Source: CAD feature listing. Evaluate the final solid. Frame: model axes, mm. A direction names the side the tool comes from. Coordinates: 2 decimals unless noted, no trailing zeros. Loops run counter-clockwise (first coordinate to the right, second up) from the corner with the lowest first, then second, coordinate; pieces in that order, holes last. Notation, with made-up numbers: (21.5, 6) -> (48.5, 6) arc R18 cw to (48.5, 14) -> close; hole circle Ø10 at (-34.75, -34.75). An arc over 180 degrees is marked (long way). Answer as a JSON object with one key per item and string values. Group by question number.
from build123d import *

# Parameters (mm, degrees)
F1_DEPTH = 20
F2_T     = -3
F4_DEPTH = 20
F6_D     = 4.3
F6_DEPTH = 5
F6_TIP   = 1.2918503309


with BuildPart() as f1:
    # F0 (on Top) → F1 (new body)
    with BuildSketch(Plane.XY):
        Polygon((0, 100), (0, 0), (173.2050807569, 0), align=None)
    extrude(amount=F1_DEPTH)

    # F2
    f2_openings = [f1.faces().sort_by_distance(p)[0] for p in [
        (57.735027, 33.333333, 20),
        (57.735027, 33.333333, 0),
    ]]
    offset(amount=F2_T, openings=f2_openings)

    # F3 (on face) → F4 (join)
    with BuildSketch(Plane.XY.offset(20)):
        Polygon((86.6025403784, 3), (86.6025403784, 46.5358983849), (83.6025403784, 48.2679491924), (83.6025403784, 3), align=None)
    extrude(amount=-F4_DEPTH)

    # F6
    with Locations(Plane.XZ):
        with Locations((30, 10), (123.2050807569, 10)):
            Hole(F6_D / 2, depth=F6_DEPTH)
            with Locations((0, 0, -(F6_DEPTH + F6_TIP / 2))):  # 118° drill point
                Cone(0, F6_D / 2, F6_TIP, mode=Mode.SUBTRACT)


solid = f1.part
1. Section query D-D on z = 10. Return loops of the section in (x, y), then the cut area to 3 significant figures.
2. Section query B-B on x = 141. Return loops of the section in (y, z).
3. Mould query, pull axis X, two halves, no side actions, for faces 4 (the face through (54, 2, 0)), 5 (the face through (43.865, 71.21, 9.86)), 6 (the face through (0, 51, 10)), 7 (the face through (3, 50, 10)). Classes: pulls with the +X half, pulls with the -X half, needs draft (parallel to the pull), parting line crosses it, or undercut.
4. Section query C-C on z = 18. Return loops of the section in (x, y), then the cut area to 3 significant figures.
5. Ray query, L1, parallel to Z at x = 30, y = 0.7; L2, parallel to X at y = 14.5, z = 14; L3, parallel to X at y = 31, z = 8.25. Return the intervals inside material, ascending.
6. Pin query (flat end, axial travel): pin 1 Ø1.5 at (x, y) = (23, 88) entering from -Z; pin 2 Ø6 at (y, z) = (16.5, 11.5) entering from +X; pin 3 Ø3.5 at (x, z) = (30, 10) entering from -Y (3 decimals); pin 4 Ø6 at (y, z) = (34.5, 9) entering from +X. Return the tip coordinate at first contact, or that it passes through.
7. Reachability of faces 1 (the face through (125.353, 1.521, 10.095)), 2 (the face through (85, 0, 10)), 3 (the face through (43, 3, 10)) from +Z, -Z, +X, -X, +Y, -Y: full face, straight path, thin tool, end or side. Return the list, or none.
8. Section query A-A on y = 23. Return loops of the section in (x, z).
Solved:
{
 "1": {"outline": "(0, 0) -> (27.85, 0) -> (27.85, 3) -> (3, 3) -> (3, 94.8) -> (83.6, 48.27) -> (83.6, 3) -> (32.15, 3) -> (32.15, 0) -> (121.06, 0) -> (121.06, 3) -> (86.6, 3) -> (86.6, 46.54) -> (162.01, 3) -> (125.36, 3) -> (125.36, 0) -> (173.21, 0) -> (0, 100) -> close", "area": "1,470 mm^2"},
 "2": {"outline": "(0, 0) -> (3, 0) -> (3, 20) -> (0, 20) -> close; (15.13, 0) -> (18.59, 0) -> (18.59, 20) -> (15.13, 20) -> close"},
 "3": {"face 4": "needs draft", "face 5": "undercut", "face 6": "pulls with the -X half", "face 7": "undercut"},
 "4": {"outline": "(0, 0) -> (173.21, 0) -> (0, 100) -> close; hole (3, 3) -> (83.6, 3) -> (83.6, 48.27) -> (3, 94.8) -> close; hole (86.6, 3) -> (162.01, 3) -> (86.6, 46.54) -> close", "area": "1,490 mm^2"},
 "5": {"L1": "0 to 7.85, 12.15 to 20", "L2": "0 to 3, 83.6 to 86.6, 142.09 to 148.09", "L3": "0 to 3, 83.6 to 86.6, 113.51 to 119.51"},
 "6": {"pin 1": "through", "pin 2": "x = 149.82", "pin 3": "y = 78.205", "pin 4": "x = 118.65"},
 "7": {"face 1": "-Y", "face 2": "+Z, -Z, +X, -X, -Y", "face 3": "+Z, -Z"},
 "8": {"outline": "(0, 0) -> (3, 0) -> (3, 20) -> (0, 20) -> close; (83.6, 0) -> (86.6, 0) -> (86.6, 20) -> (83.6, 20) -> close; (127.37, 0) -> (133.37, 0) -> (133.37, 20) -> (127.37, 20) -> close"}
}
